from build123d import *

# Parameters (mm, degrees)
F1_DEPTH        = 5
F4_D            = 11
F4_DEPTH        = 57.15
F4_CSINK_D      = 22.4
F4_CSINK_ANGLE  = 90
F4_TIP          = 3.3047334047
F5_D            = 5.5
F5_DEPTH        = 57.15
F5_CSINK_D      = 11.2
F5_CSINK_ANGLE  = 90
F5_TIP          = 1.6523667023
F7_DEPTH        = 2
F7_COPIES_COUNT = 6


# Not quite as in the source:
# - a pattern or mirror of a feature is missing from the dataset's text; its kind, count and spacing are read off the source's solid


with BuildPart() as f1:
    # F0 (on Top) → F1 (new body, symmetric)
    with BuildSketch(Plane.XY):
        Polygon((28.8675134595, 50), (-28.8675134595, 50), (-57.735026919, 0), (-28.8675134595, -50), (28.8675134595, -50), (57.735026919, 0), align=None)
    extrude(amount=F1_DEPTH, both=True)

    # F4
    with Locations(Plane.XY.offset(5)):
        with Locations((0, 0)):
            CounterSinkHole(F4_D / 2, F4_CSINK_D / 2, depth=F4_DEPTH, counter_sink_angle=F4_CSINK_ANGLE)
            with Locations((0, 0, -(F4_DEPTH + F4_TIP / 2))):  # 118° drill point
                Cone(0, F4_D / 2, F4_TIP, mode=Mode.SUBTRACT)

    # F5
    with Locations(Plane.XY.offset(5)):
        with Locations((21.6506350946, 37.5), (43.3012701892, 0), (21.6506350946, -37.5), (-21.6506350946, -37.5), (-43.3012701892, 0), (-21.6506350946, 37.5)):
            CounterSinkHole(F5_D / 2, F5_CSINK_D / 2, depth=F5_DEPTH, counter_sink_angle=F5_CSINK_ANGLE)
            with Locations((0, 0, -(F5_DEPTH + F5_TIP / 2))):  # 118° drill point
                Cone(0, F5_D / 2, F5_TIP, mode=Mode.SUBTRACT)

    # F6 (on Top) → F7 (cut, symmetric)
    with BuildSketch(Plane.XY):
        with BuildLine():
            ThreePointArc((-19.2690652342, -38.875), (-18.9943390723, -38.211752374), (-18.9006350946, -37.5))
            ThreePointArc((-18.9006350946, -37.5), (-20.9388827206, -34.8437039777), (-24.032204955, -36.125))
            ThreePointArc((-24.032204955, -36.125), (-23.0256350946, -39.8815698604), (-19.2690652342, -38.875))
        make_face()
        with BuildLine():
            ThreePointArc((-19.2690652342, -38.875), (-23.0256350946, -39.8815698604), (-24.032204955, -36.125))
            Line((-24.032204955, -36.125), (-30.4552266998, -47.25))
            Line((-30.4552266998, -47.25), (-28.8675134595, -50))
            Line((-28.8675134595, -50), (-25.6920869789, -50))
            Line((-25.6920869789, -50), (-19.2690652342, -38.875))
        make_face()
    f7 = extrude(amount=F7_DEPTH, both=True, mode=Mode.SUBTRACT)

    # F7_copies: F7 ×6 about axis
    f7_copies_axis = Axis((0, 0, 0), (0, 0, 1))
    for i in range(1, F7_COPIES_COUNT):
        add(f7.rotate(f7_copies_axis, i * 360 / F7_COPIES_COUNT), mode=Mode.SUBTRACT)


solid = f1.part
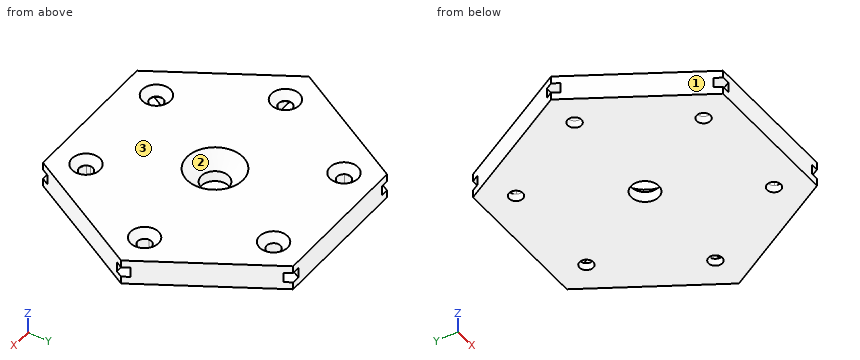
Verification items for the finished model (mm, model axes). Face numbers are marked on the shaded views. Give positions to 0.01 mm unless a question says otherwise; leave off trailing zeros. Order: outer loops, then holes, each group sorted by start corner. A loop starts at its lowest first (then second) coordinate and runs counter-clockwise, first axis right, second up. Notation, with made-up numbers: (26, -7) -> (82, -7) arc R26 cw to (82, 22) -> close; hole circle Ø10 at (16.5, 14). An arc over 180 degrees is marked (long way). Answer as CSV lines item,"result".
Q1. Scan lines: probe 1 along Y at (x, z) = (23.5, -3.5); probe 2 along Y at (x, z) = (23.5, 4); probe 3 along X at (y, z) = (0, 2.1). Record each from-to range of solid material in increasing order.
Solutions:
probe 1,"y = -50 to -39.54, -35.46 to 35.46, 39.54 to 50"
probe 2,"y = -50 to -41.71, -33.29 to 33.29, 41.71 to 50"
probe 3,"x = -57.74 to -46.05, -40.55 to -8.3, 8.3 to 40.55, 46.05 to 57.74"
Q2. Release check for a two-part mould opening along X. For the marked faces 1, 2 and 3 record: +X half, -X half, draft (parallel to the pull), parting line (faces both ways), or undercut.
Solutions:
face 1,"-X half"
face 2,"undercut"
face 3,"draft"
Q3. Depth check by flat-ended pin: pin 1 (3 mm diameter, centred on y = 18.5, z = 2.5, fed in from +X); pin 2 (3 mm diameter, centred on x = -50, z = 0, fed in from -Y); pin 3 (1.2 mm diameter, centred on x = 47, z = -0.5, fed in from +Y). Enter the tip coordinate at first touch or a pass-through.
Solutions:
pin 1,"stops at x = 47.92"
pin 2,"stops at y = -16"
pin 3,"stops at y = 19.63"
Q4. Sectioned sample at B-B on y = 37.5. Record the cut outline in (x, z), plus the area to 3 significant figures.
Solutions:
outline,"(-36.08, -5) -> (-24.4, -5) -> (-24.4, -2) -> (-24.83, -2) -> (-24.83, 2) -> (-24.4, 2) -> (-24.4, 2.15) -> (-27.25, 5) -> (-36.08, 5) -> close; (-18.9, -5) -> (18.9, -5) -> (18.9, 2.15) -> (16.05, 5) -> (-16.05, 5) -> (-18.9, 2.15) -> close; (24.4, -5) -> (36.08, -5) -> (36.08, 5) -> (27.25, 5) -> (24.4, 2.15) -> (24.4, 2) -> (24.83, 2) -> (24.83, -2) -> (24.4, -2) -> close"
area,"592 mm²"
Q5. Sectioned sample at D-D on y = -22.5. Record the cut outline in (x, z).
Solutions:
outline,"(-44.74, -5) -> (44.74, -5) -> (44.74, 5) -> (-44.74, 5) -> close"
Q6. Sectioned sample at A-A on x = 0. Record the cut outline in (y, z).
Solutions:
outline,"(-50, -5) -> (-5.5, -5) -> (-5.5, -0.7) -> (-11.2, 5) -> (-50, 5) -> close; (5.5, -5) -> (50, -5) -> (50, 5) -> (11.2, 5) -> (5.5, -0.7) -> close"
Q7. Sectioned sample at C-C on z = 3.5. Record the cut outline in (x, y).
Solutions:
outline,"(-57.74, 0) -> (-28.87, -50) -> (28.87, -50) -> (57.74, 0) -> (28.87, 50) -> (-28.87, 50) -> close; hole circle Ø8.2 at (-43.3, 0); hole circle Ø8.2 at (-21.65, -37.5); hole circle Ø8.2 at (-21.65, 37.5); hole circle Ø19.4 at (0, 0); hole circle Ø8.2 at (21.65, -37.5); hole circle Ø8.2 at (21.65, 37.5); hole circle Ø8.2 at (43.3, 0)"
